Check sheet for the modelled part. Datum: model origin and axes. Units: mm. Face numbers are marked on the shaded views. Coordinates: 2 decimals unless noted, no trailing zeros. Loops run counter-clockwise (first coordinate to the right, second up) from the corner with the lowest first, then second, coordinate; pieces in that order, holes last. Notation, with made-up numbers: M -40,-21.75 L -22,-21.75 A22 cw -22,17.25 Z; hole C 55,88 d8. An arc over 180 degrees is marked long. Write each question's results on one line, items separated by ' | '. Start each with the question number.
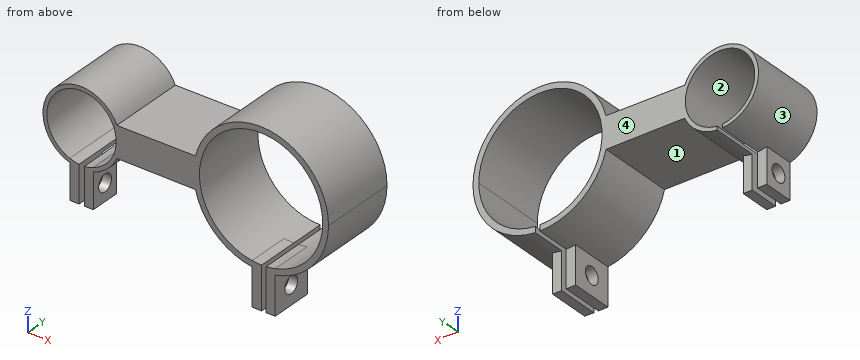
from build123d import *

# Parameters (mm, degrees)
F0_R      = 12.7
F0_R_2    = 11.43
F1_DEPTH  = 25.4
F3_R      = 20.32
F4_DEPTH  = 25.4
F5_W      = 3.0645749275
F5_H      = 25.4
F6_DEPTH  = 10.16
F8_DEPTH  = 30.226
F9_DEPTH  = 25.4
F10_R     = 2.794
F11_DEPTH = 25.4
F13_W     = 3.175
F13_H     = 35.56
F14_DEPTH = 13.97
F15_R     = 2.794
F16_DEPTH = 25.4
F18_DEPTH = 30.734
F20_DEPTH = 40.64
F22_DEPTH = 25.4


with BuildPart() as f1:
    # F0 (on Front) → F1 (new body)
    with BuildSketch(Plane.XZ):
        Circle(F0_R)
        Circle(F0_R_2, mode=Mode.SUBTRACT)
    extrude(amount=F1_DEPTH)

    # F5 (on offset) → F6 (join)
    with BuildSketch(Plane.XZ.offset(25.4)):
        with Locations((-2.327306883, -11.0291545425)):
            Rectangle(F5_W, F5_H)
        Polygon((3.894138498, 1.6708454575), (0.9391864802, 1.6708454575), (0.9391864802, -23.7291545425), (3.894138498, -23.7291545425), (3.894138498, -11.0291545425), align=None)
    extrude(amount=-F6_DEPTH)

    # F7 (on face) → F8 (cut)
    with BuildSketch(Plane.XZ.offset(25.4)):
        Polygon((-3.8595943467, 6.5400209701), (-3.8595943467, -10.7586445001), (-0.7950194192, -10.7537217399), (0.9391864802, -10.7509360094), (3.894138498, -10.7461893413), (3.894138498, 6.8227690223), align=None)
        Polygon((0.9391864802, -10.7509360094), (-0.7950194192, -10.7537217399), (-0.7950194192, -12.6750914838), (0.9391864802, -12.6652251759), (0.9391864802, -11.3913488558), align=None)
    extrude(amount=-F8_DEPTH, mode=Mode.SUBTRACT)

    # F7 (on face) → F9 (cut)
    with BuildSketch(Plane.XZ.offset(25.4)):
        Polygon((-3.8595943467, 6.5400209701), (-3.8595943467, -10.7586445001), (-0.7950194192, -10.7537217399), (0.9391864802, -10.7509360094), (3.894138498, -10.7461893413), (3.894138498, 6.8227690223), align=None)
        Polygon((0.9391864802, -10.7509360094), (-0.7950194192, -10.7537217399), (-0.7950194192, -12.6750914838), (0.9391864802, -12.6652251759), (0.9391864802, -11.3913488558), align=None)
    extrude(amount=-F9_DEPTH, mode=Mode.SUBTRACT)

    # F10 (on face) → F11 (cut)
    with BuildSketch(Plane(origin=(-3.8595943467, 0, 0), x_dir=(0, -1, 0), z_dir=(-1, 0, 0))):
        with Locations((20.32, -17.914237003)):
            Circle(F10_R)
    extrude(amount=-F11_DEPTH, mode=Mode.SUBTRACT)


with BuildPart() as f4:
    # F3 (on offset) → F4 (new body)
    with BuildSketch(Plane.XZ.offset(25.4)):
        with BuildLine():
            Line((37.5699403561, 5.2842361421), (10.6034887032, 5.0843427817))
            ThreePointArc((10.6034887032, 5.0843427817), (11.5328465432, 2.6263680661), (11.8205691299, 0.0143647333))
            Line((11.8205691299, 0.0143647333), (36.950101903, 0.0449029444))
            ThreePointArc((36.950101903, 0.0449029444), (37.1040026209, 2.6830272873), (37.5699403561, 5.2842361421))
        make_face()
        with BuildLine():
            ThreePointArc((81.4000854922, 0.0719114545), (61.799611578, 22.1414036966), (37.5699403561, 5.2842361421))
            Line((37.5699403561, 5.2842361421), (38.7200076161, 5.2927612092))
            ThreePointArc((38.7200076161, 5.2927612092), (37.3247254516, 0.1119146147), (38.6803581082, -5.079447813))
            Line((38.6803581082, -5.079447813), (37.5553231739, -5.079447813))
            ThreePointArc((37.5553231739, -5.079447813), (61.7684816706, -22.0012605256), (81.4000854922, 0.0719114545))
        make_face()
        with Locations((59.1750854922, 0.0719114545)):
            Circle(F3_R, mode=Mode.SUBTRACT)
        with BuildLine():
            Line((38.7200076161, 5.2927612092), (37.5699403561, 5.2842361421))
            ThreePointArc((37.5699403561, 5.2842361421), (37.1040026209, 2.6830272873), (36.950101903, 0.0449029444))
            ThreePointArc((36.950101903, 0.0449029444), (37.1034933748, -2.5348962497), (37.5553231739, -5.079447813))
            Line((37.5553231739, -5.079447813), (38.6803581082, -5.079447813))
            ThreePointArc((38.6803581082, -5.079447813), (37.3247254516, 0.1119146147), (38.7200076161, 5.2927612092))
        make_face()
        with BuildLine():
            Line((36.950101903, 0.0449029444), (11.8205691299, 0.0143647333))
            ThreePointArc((11.8205691299, 0.0143647333), (11.4383828548, -2.6236056978), (10.4021426077, -5.079447813))
            Line((10.4021426077, -5.079447813), (37.5553231739, -5.079447813))
            ThreePointArc((37.5553231739, -5.079447813), (37.1034933748, -2.5348962497), (36.950101903, 0.0449029444))
        make_face()
    extrude(amount=-F4_DEPTH)


with BuildPart() as f1_1:
    add(f1.part)

    # F12: union F4
    add(f4.part)

    # F13 (on face) → F14 (join)
    with BuildSketch(Plane.XZ.offset(25.4)):
        Polygon((63.8311807601, 1.2001052282), (60.8582296082, 1.2001052282), (60.8582296082, -34.3598947718), (63.8311807601, -34.3598947718), (63.8311807601, -21.6598947718), align=None)
        with Locations((57.7986807601, -16.5798947718)):
            Rectangle(F13_W, F13_H)
    extrude(amount=-F14_DEPTH)

    # F15 (on face) → F16 (cut)
    with BuildSketch(Plane.YZ.offset(63.8311807601)):
        with Locations((-18.415, -28.0098947718)):
            Circle(F15_R)
    extrude(amount=-F16_DEPTH, mode=Mode.SUBTRACT)

    # F17 (on face) → F18 (cut)
    with BuildSketch(Plane.XZ.offset(25.4)):
        with BuildLine():
            ThreePointArc((63.8311807601, -19.7074509431), (58.3136851955, 20.3736451127), (56.2111807601, -20.0307666939))
            Line((56.2111807601, -20.0307666939), (56.2111807601, 1.2001052282))
            Line((56.2111807601, 1.2001052282), (59.3861807601, 1.2001052282))
            Line((59.3861807601, 1.2001052282), (60.8582296082, 1.2001052282))
            Line((60.8582296082, 1.2001052282), (63.8311807601, 1.2001052282))
            Line((63.8311807601, 1.2001052282), (63.8311807601, -19.7074509431))
        make_face()
        with BuildLine():
            Line((56.2111807601, 1.2001052282), (56.2111807601, -20.0307666939))
            ThreePointArc((56.2111807601, -20.0307666939), (57.7944413181, -20.2011302922), (59.3861807601, -20.2469920294))
            Line((59.3861807601, -20.2469920294), (59.3861807601, 1.2001052282))
            Line((59.3861807601, 1.2001052282), (56.2111807601, 1.2001052282))
        make_face()
        with BuildLine():
            ThreePointArc((60.8582296082, -20.1782595543), (62.3534347774, -19.9979788248), (63.8311807601, -19.7074509431))
            Line((63.8311807601, -19.7074509431), (63.8311807601, 1.2001052282))
            Line((63.8311807601, 1.2001052282), (60.8582296082, 1.2001052282))
            Line((60.8582296082, 1.2001052282), (60.8582296082, -20.1782595543))
        make_face()
        with BuildLine():
            ThreePointArc((60.8582296082, -20.1782595543), (60.1228284685, -20.2259747224), (59.3861807601, -20.2469920294))
            Line((59.3861807601, -20.2469920294), (59.3861807601, -22.1520860209))
            Line((59.3861807601, -22.1520860209), (60.8582296082, -22.0892629477))
            Line((60.8582296082, -22.0892629477), (60.8582296082, -20.1782595543))
        make_face()
        with BuildLine():
            Line((59.3861807601, 1.2001052282), (59.3861807601, -20.2469920294))
            ThreePointArc((59.3861807601, -20.2469920294), (60.1228284685, -20.2259747224), (60.8582296082, -20.1782595543))
            Line((60.8582296082, -20.1782595543), (60.8582296082, 1.2001052282))
            Line((60.8582296082, 1.2001052282), (59.3861807601, 1.2001052282))
        make_face()
        Polygon((60.8582296082, -22.0892629477), (59.3861807601, -22.1520860209), (59.3861807601, -22.3753936589), (60.8582296082, -22.3753936589), align=None)
    extrude(amount=-F18_DEPTH, mode=Mode.SUBTRACT)

    # F19 (on face) → F20 (cut)
    with BuildSketch(Plane.XZ.offset(25.4)):
        with BuildLine():
            Line((-3.8612207101, -9.7461815458), (-3.8595943467, -10.7586445001))
            ThreePointArc((-3.8595943467, -10.7586445001), (0.0185050029, -11.5199534125), (3.894138498, -10.7461893413))
            Line((3.894138498, -10.7461893413), (3.894138498, -9.7337237745))
            Line((3.894138498, -9.7337237745), (-3.8612207101, -9.7461815458))
        make_face()
    extrude(amount=-F20_DEPTH, mode=Mode.SUBTRACT)

    # F21 (on face) → F22 (cut)
    with BuildSketch(Plane.XZ.offset(25.4)):
        Polygon((0.9391864802, -11.4767284574), (-0.7950194192, -11.4886898794), (-0.7950194192, -13.0471941084), (0.9391864802, -13.0471941084), align=None)
    extrude(amount=-F22_DEPTH, mode=Mode.SUBTRACT)


solid = f1_1.part
1) Gauge pin test, flat ends, axial feed: P1, Ø1.5, axis at x = 37, z = -10.5, coming from the -Y side; P2, Ø1.5, axis at x = 62.5, z = -29, coming from the +Y side; P3, Ø2.5, axis at x = 3, z = -16, coming from the +Y side; P4, Ø2, axis at x = 35.5, y = -10, coming from the +Z side. Record the tip position at first contact, or that the pin passes through.
2) Release check for a two-part mould opening along Z. For the marked faces 1, 2, 3 and 4 record: +Z half, -Z half, draft (parallel to the pull), parting line (faces both ways), or undercut.
3) Section check C-C (y = -19.75). Give the number of separate pieces and of enclosed holes in the cut face, then the cut area to 3 significant figures.
4) Thickness scan on probe 1 along X at (y, z) = (-21, 0.5); probe 2 along X at (y, z) = (-9, 11.5); probe 3 along Z at (x, y) = (-2.55, -20.32). Record the ranges inside material, lowest first.
5) Section check B-B (z = -2). Enter the section's corners in (x, y).
6) Section check A-A (x = 46). Enter the section's corners in (y, z), then the cut area to 3 significant figures.
Return value:
1) P1: passes through | P2: stops at y = -11.43 | P3: stops at y = -15.24 | P4: stops at z = 5.28
2) face 1: -Z half | face 2: undercut | face 3: parting line | face 4: draft
3) separate pieces: 5 | enclosed holes: 0 | area: 681 mm2
4) probe 1: x = -12.69 to -11.42, 11.42 to 38.86, 79.49 to 81.4 | probe 2: x = -5.39 to 5.39, 40.11 to 42.37, 75.98 to 78.24 | probe 3: z = -23.73 to -20.71, -15.12 to -11.19, 11.14 to 12.44
5) outline: M -12.54,-25.4 L -11.25,-25.4 L -11.25,0 L -12.54,0 Z; M 11.25,-25.4 L 38.96,-25.4 L 38.96,0 L 11.25,0 Z; M 79.39,-25.4 L 81.3,-25.4 L 81.3,0 L 79.39,0 Z
6) outline: M -25.4,-17.83 L 0,-17.83 L 0,-15.4 L -25.4,-15.4 Z; M -25.4,15.54 L 0,15.54 L 0,17.97 L -25.4,17.97 Z | area: 123 mm2
